Geometry: final body of the model. Coordinates: model frame, mm. Face numbers are marked on the shaded views. Coordinates: 2 decimals unless noted, no trailing zeros. Order: outer loops, then holes, each group sorted by start corner. A loop starts at its lowest first (then second) coordinate and runs counter-clockwise, first axis right, second up. Notation, with made-up numbers: (57, 10) -> (101, 10) arc R19 cw to (101, 41) -> close; hole circle Ø10 at (-38, -22). An arc over 180 degrees is marked (long way). Use CSV: the item, a comma, the result in double quotes. Start each with the question number.
from build123d import *

# Parameters (mm, degrees)
SKETCH1_R           = 32
SKETCH1_R_2         = 30
BOSS_EXTRUDE1_DEPTH = 10
BOSS_EXTRUDE2_START = 100
SKETCH1_3_R         = 32
SKETCH1_3_R_2       = 30
BOSS_EXTRUDE2_DEPTH = 100
FILLET1_R           = 5
FILLET2_R           = 5
SKETCH2_R           = 2.5
BOSS_EXTRUDE3_DEPTH = 2
CHAMFER1_SIZE       = 2.5
CHAMFER1_SIZE_2     = 6.868693549


with BuildPart() as part:
    # Sketch1 → Boss-Extrude1 (new body)
    # profile 1 of 2: a face of its own
    with BuildSketch(Plane(origin=(0, 0, 0), x_dir=(1, 0, 0), z_dir=(0, 1, 0))):
        with Locations(Location((0, 0, 0), (0, 0, 270))):
            Circle(SKETCH1_R)
        Circle(SKETCH1_R_2, mode=Mode.SUBTRACT)
    # profile 2 of 2: a face of its own
    with BuildSketch(Plane(origin=(0, 0, 0), x_dir=(1, 0, 0), z_dir=(0, 1, 0))):
        Circle(SKETCH1_R_2)
    extrude(amount=-BOSS_EXTRUDE1_DEPTH)

    # Sketch1<3> → Boss-Extrude2 (add)
    with BuildSketch(Plane(origin=(0, 0, 0), x_dir=(1, 0, 0), z_dir=(0, 1, 0)).offset(BOSS_EXTRUDE2_START)):
        with Locations(Location((0, 0, 0), (0, 0, 270))):
            Circle(SKETCH1_3_R)
        with Locations(Location((0, 0, 0), (0, 0, 270))):
            Circle(SKETCH1_3_R_2, mode=Mode.SUBTRACT)
    extrude(amount=-BOSS_EXTRUDE2_DEPTH)

    # Fillet1
    fillet1_edges = [part.edges().sort_by_distance(p)[0] for p in [
        (0, 0, -30),
    ]]
    fillet(fillet1_edges, radius=FILLET1_R)

    # Fillet2
    fillet2_edges = [part.edges().sort_by_distance(p)[0] for p in [
        (0, -10, -32),
    ]]
    fillet(fillet2_edges, radius=FILLET2_R)

    # Sketch2 → Boss-Extrude3 (add)
    # profile 1 of 3: a face of its own
    with BuildSketch(Plane.XZ.offset(10)):
        with BuildLine():
            Line((-16.887495374, -12.25), (16.887495374, -12.25))
            ThreePointArc((16.887495374, -12.25), (19.052558883, -11), (19.052558883, -8.5))
            Line((19.052558883, -8.5), (2.165063509, 20.75))
            ThreePointArc((2.165063509, 20.75), (0, 22), (-2.165063509, 20.75))
            Line((-2.165063509, 20.75), (-19.052558883, -8.5))
            ThreePointArc((-19.052558883, -8.5), (-19.052558883, -11), (-16.887495374, -12.25))
        make_face()
        Polygon((-16.887495374, -9.75), (16.887495374, -9.75), (0, 19.5), align=None, mode=Mode.SUBTRACT)
    # profile 2 of 3: a face of its own
    with BuildSketch(Plane.XZ.offset(10)):
        with BuildLine():
            Line((-2.5, 12), (-2.5, 0))
            ThreePointArc((-2.5, 0), (0, -2.5), (2.5, 0))
            Line((2.5, 0), (2.5, 12))
            ThreePointArc((2.5, 12), (0, 14.5), (-2.5, 12))
        make_face()
    # profile 3 of 3: a face of its own
    with BuildSketch(Plane.XZ.offset(10)):
        with Locations(Location((0, -6, 0), (0, 0, 90))):
            Circle(SKETCH2_R)
    extrude(amount=BOSS_EXTRUDE3_DEPTH)

    # Chamfer1
    # the kernel refuses this chamfer: 6.868693549, 2.5 mm, written as the material it takes off along each edge
    with BuildSketch(Plane(origin=(0, 100, 0), x_dir=(0, 0, 1), z_dir=(-1, 0, 0))) as chamfer1_piece_1:
        Polygon((30 + CHAMFER1_SIZE, 0), (30, -CHAMFER1_SIZE_2), (30, 0), align=None)
    revolve(axis=Axis((0, 100, 0), (0, 1, 0)), mode=Mode.SUBTRACT)


solid = part.part
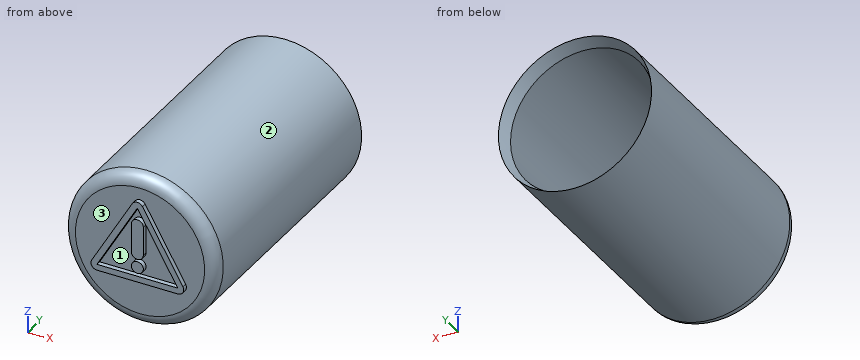
(1) Line query: line 1 (X direction, y = 40, z = 0); line 2 (Y direction, x = -8, z = -8); line 3 (X direction, y = 42, z = -24). Output: solid intervals per line, ascending. Write a range as from..to.
(2) Section A-A (y = 66.5). Return loops of the section in (x, z), then the cut area to 3 significant figures.
(3) Mould query, pull axis X, two halves, no side actions, for the marked faces 1, 2 and 3. Classes: pulls with the +X half, pulls with the -X half, needs draft (parallel to the pull), parting line crosses it, or undercut.
(4) First-contact query: pin 1 (1 mm diameter, centred on y = 68, z = -13, fed in from -X); pin 2 (25 mm diameter, centred on x = -3.5, z = -12, fed in from +Y); pin 3 (6 mm diameter, centred on x = -13.5, y = 16.5, fed in from +Z); pin 4 (23.5 mm diameter, centred on x = 6.5, z = -1.5, fed in from -Y). Flat tips, straight axial feed; report the tip coordinate or a pass-through.
Check sheet entries:
1,line 1,"x = -32..-30, 30..32"
1,line 2,"y = -10..0"
1,line 3,"x = -21.17..-18, 18..21.17"
2,outline,"circle Ø64 at (0, 0); hole circle Ø60 at (0, 0)"
2,area,"390 mm^2"
3,face 1,"undercut"
3,face 2,"parting line crosses it"
3,face 3,"needs draft"
4,pin 1,"stops at x = -29.46"
4,pin 2,"stops at y = 0"
4,pin 3,"stops at z = 30.23"
4,pin 4,"stops at y = -12"
